Source: CAD feature listing. Evaluate the final solid. Frame: model axes, mm. A direction names the side the tool comes from. Round coordinates to 2 decimals unless told otherwise and drop trailing zeros. Order: outer loops, then holes, each group sorted by start corner. A loop starts at its lowest first (then second) coordinate and runs counter-clockwise, first axis right, second up. Notation, with made-up numbers: (4, -25.5) - (11, -25.5) arc R27 cw to (11, 3.5) - close; hole circle Ø1 at (20, 63.25). An arc over 180 degrees is marked (long way). Use one line per item in the form item = value. Start each with the question number.
Q1. Cut plane C-C, the plane z = -0.5. Return the cut outline in (x, y).
Q2. Cut plane D-D, the plane x = -6.25. Return the cut outline in (y, z).
Q3. Pin query (flat end, axial travel): pin 1 Ø1.5 at (x, z) = (-3.5, 0.5) entering from -Y; pin 2 Ø1 at (x, z) = (-4, 0.5) entering from -Y; pin 3 Ø3 at (y, z) = (-7, 1) entering from +X. Return the tip coordinate at first contact, or that it passes through.
Q4. Set-up query: faces 1 (the cylindrical face through (2.003, 0.631, -0.05)), 2 (the flat face through (-7, -5, 1.4)). Return all of +Z, -Z, +X, -X, +Y, -Y with unobstructed straight access to the full face (end or side cutting, diameter ignored); none if empty.
Q5. Ray query, line 1 (Z direction, x = -2.25, y = 8.5); line 2 (Y direction, x = 0, z = -0.75); line 3 (Y direction, x = -1.5, z = 0.75). Return the intervals inside material, ascending. Write a range as [from, to].
Q6. Cut plane A-A, the plane x = 0. Return the cut outline in (y, z).
Q7. Draft query along Z for faces 3 (the cylindrical face through (10, 3.2, 2.5)), 4 (the flat face through (-0.1, 2.5, -3.6)), 5 (the cylindrical face through (7.964, 2.508, -0.02)), 6 (the flat face through (-0.1, 2.5, 3.6)). Return one class per face: released by +Z, released by -Z, zero draft, split by the parting line, or undercut.
from build123d import *

# Parameters (mm, degrees)
F_01_START                           = -1.4
S01_GROOVE_ROOT_AND_AXLE_BORE_R      = 8.35
S01_GROOVE_ROOT_AND_AXLE_BORE_R_2    = 2.1
F_01_GROOVE_ROOT_AND_AXLE_BORE_DEPTH = 2.8
F_02_START                           = -3.6
S02_RETAINING_FLANGE_3_6_R           = 10.5
S02_RETAINING_FLANGE_3_6_R_2         = 2.1
F_02_RETAINING_FLANGE_3_6_DEPTH      = 2.2
F_03_START                           = 1.4
S03_RETAINING_FLANGE_1_4_R           = 10.5
S03_RETAINING_FLANGE_1_4_R_2         = 2.1
F_03_RETAINING_FLANGE_1_4_DEPTH      = 2.2


with BuildPart() as part:
    # S01 - Groove root and axle bore → 01 - Groove root and axle bore (new body)
    with BuildSketch(Plane.XY.offset(F_01_START)):
        Circle(S01_GROOVE_ROOT_AND_AXLE_BORE_R)
        Circle(S01_GROOVE_ROOT_AND_AXLE_BORE_R_2, mode=Mode.SUBTRACT)
    extrude(amount=F_01_GROOVE_ROOT_AND_AXLE_BORE_DEPTH)

    # S02 - Retaining flange -3.6 → 02 - Retaining flange -3.6 (add)
    with BuildSketch(Plane.XY.offset(F_02_START)):
        Circle(S02_RETAINING_FLANGE_3_6_R)
        Circle(S02_RETAINING_FLANGE_3_6_R_2, mode=Mode.SUBTRACT)
    extrude(amount=F_02_RETAINING_FLANGE_3_6_DEPTH)

    # S03 - Retaining flange 1.4 → 03 - Retaining flange 1.4 (add)
    with BuildSketch(Plane.XY.offset(F_03_START)):
        Circle(S03_RETAINING_FLANGE_1_4_R)
        Circle(S03_RETAINING_FLANGE_1_4_R_2, mode=Mode.SUBTRACT)
    extrude(amount=F_03_RETAINING_FLANGE_1_4_DEPTH)


solid = part.part
Completed:
q1.outline = circle Ø16.7 at (0, 0); hole circle Ø4.2 at (0, 0)
q2.outline = (-8.44, -3.6) - (8.44, -3.6) - (8.44, -1.4) - (5.54, -1.4) - (5.54, 1.4) - (8.44, 1.4) - (8.44, 3.6) - (-8.44, 3.6) - (-8.44, 1.4) - (-5.54, 1.4) - (-5.54, -1.4) - (-8.44, -1.4) - close
q3.pin_1 = -7.88
q3.pin_2 = -7.58
q3.pin_3 = 8.91
q4.face_1 = +Z, -Z
q4.face_2 = none
q5.line_1 = [-3.6, -1.4], [1.4, 3.6]
q5.line_2 = [-8.35, -2.1], [2.1, 8.35]
q5.line_3 = [-8.21, -1.47], [1.47, 8.21]
q6.outline = (-10.5, -3.6) - (-2.1, -3.6) - (-2.1, 3.6) - (-10.5, 3.6) - (-10.5, 1.4) - (-8.35, 1.4) - (-8.35, -1.4) - (-10.5, -1.4) - close; (2.1, -3.6) - (10.5, -3.6) - (10.5, -1.4) - (8.35, -1.4) - (8.35, 1.4) - (10.5, 1.4) - (10.5, 3.6) - (2.1, 3.6) - close
q7.face_3 = zero draft
q7.face_4 = released by -Z
q7.face_5 = undercut
q7.face_6 = released by +Z
